Read the model definition and answer for the solid it produces. Units are mm, in the model's axes. A direction names the side the tool comes from. Round coordinates to 2 decimals unless told otherwise and drop trailing zeros. Order: outer loops, then holes, each group sorted by start corner. A loop starts at its lowest first (then second) coordinate and runs counter-clockwise, first axis right, second up. Notation, with made-up numbers: (55, 75.5) - (60, 75.5) arc R22 ccw to (60, 112.5) - close; hole circle Ø4 at (-38.5, 82). An arc over 180 degrees is marked (long way). Put each result on its own line as item: value. Start each with the question number.
Q1. For a pull along Z with two mould halves and no side action, classify faces 3 (the face through (-1, -38.1, -25)), 4 (the face through (-51.3, -9.525, -30.4)), 5 (the face through (-1, -19, 0)) as pulls with the +Z half, pulls with the -Z half, needs draft (parallel to the pull), parting line crosses it, or undercut.
Q2. Section A-A on z = -19.5 is taken. Give the vertices of the cut face in (x, y) (3 decimals), then the cut area to 3 significant figures.
Q3. Find the intervals of material crossed by line 1 along X through (y, z) = (-30.5, -26); line 2 along X through (y, z) = (-31.5, -30.5); line 3 along Z through (x, y) = (-44, -29.5), in increasing order. Write a range as from..to.
Q4. Section D-D on z = -32 is taken. Give the vertices of the cut face in (x, y) (3 decimals).
Q5. This flat-tipped pin is pushed along its axis until it touches: pin 1 Ø10 at (x, z) = (-52.5, -21) entering from -Y (3 decimals). Where does it stop, or does it pass through?
Q6. Section C-C on y = -12.5 is taken. Give the vertices of the cut face in (x, z), then the cut area to 3 significant figures.
Q7. Section B-B on x = 44 is taken. Give the vertices of the cut face in (y, z) (3 decimals), then the cut area to 3 significant figures.
Q8. Which of the six approach directions +Z, -Z, +X, -X, +Y, -Y give full straight-line access (tool end or side, diameter ignored) to faces 1 (the face through (-1, -19, -50.8)), 2 (the face through (-58.903, -23.612, -20.761))?
from build123d import *

# Parameters (mm, degrees)
F0_W     = 152.4
F0_H     = 50.8
F1_DEPTH = 38.1
F2_R     = 6.7437
F3_DEPTH = 9.525
F4_R     = 10.16
F5_DEPTH = 152.4


with BuildPart() as f1:
    # F0 (on Front) → F1 (new body)
    with BuildSketch(Plane.XZ):
        with Locations((0, -25.4)):
            Rectangle(F0_W, F0_H)
    extrude(amount=F1_DEPTH)

    # F2 (on face) → F3 (cut)
    with BuildSketch(Plane(origin=(0, 0, 0), x_dir=(-1, 0, 0), z_dir=(0, 1, 0))):
        with Locations((49.2125, -23.8125)):
            Circle(F2_R)
        with Locations((-49.2125, -23.8125)):
            Circle(F2_R)
    extrude(amount=-F3_DEPTH, mode=Mode.SUBTRACT)

    # F4 (on face) → F5 (cut)
    with BuildSketch(Plane(origin=(0, -9.525, 0), x_dir=(-1, 0, 0), z_dir=(0, 1, 0))):
        with Locations((-49.2125, -23.8125)):
            Circle(F4_R)
        with Locations((49.2125, -23.8125)):
            Circle(F4_R)
    extrude(amount=-F5_DEPTH, mode=Mode.SUBTRACT)


solid = f1.part
Findings:
1. face 3: needs draft
1. face 4: undercut
1. face 5: pulls with the +Z half
2. outline: (-76.2, -38.1) - (-58.412, -38.1) - (-58.412, -9.525) - (-54.397, -9.525) - (-54.397, 0) - (-76.2, 0) - close; (-44.028, -9.525) - (-40.013, -9.525) - (-40.013, -38.1) - (40.013, -38.1) - (40.013, -9.525) - (44.028, -9.525) - (44.028, 0) - (-44.028, 0) - close; (54.397, -9.525) - (58.412, -9.525) - (58.412, -38.1) - (76.2, -38.1) - (76.2, 0) - (54.397, 0) - close
2. area: 4,560 mm2
3. line 1: -76.2..-59.13, -39.29..39.29, 59.13..76.2
3. line 2: -76.2..-56.86, -41.56..41.56, 56.86..76.2
3. line 3: -50.8..-32.53, -15.09..0
4. outline: (-76.2, -38.1) - (-55.228, -38.1) - (-55.228, -9.525) - (-43.197, -9.525) - (-43.197, -38.1) - (43.197, -38.1) - (43.197, -9.525) - (55.228, -9.525) - (55.228, -38.1) - (76.2, -38.1) - (76.2, 0) - (-76.2, 0) - close
5. pin 1: y = -9.525
6. outline: (-76.2, -50.8) - (76.2, -50.8) - (76.2, 0) - (-76.2, 0) - close; hole circle Ø20.32 at (-49.21, -23.81); hole circle Ø20.32 at (49.21, -23.81)
6. area: 7,090 mm2
7. outline: (-38.1, -50.8) - (0, -50.8) - (0, -28.091) - (-9.525, -28.091) - (-9.525, -32.533) - (-38.1, -32.533) - close; (-38.1, -15.092) - (-9.525, -15.092) - (-9.525, -19.534) - (0, -19.534) - (0, 0) - (-38.1, 0) - close
7. area: 1,360 mm2
8. face 1: -Z, +X, -X, +Y, -Y
8. face 2: -Y
